For this review, use the dimensioned drawing (mm, ordinates from the lowest corner) and the shaded views. A direction names the side the tool comes from. Coordinates: 2 decimals unless noted, no trailing zeros. Order: outer loops, then holes, each group sorted by start corner. A loop starts at its lowest first (then second) coordinate and runs counter-clockwise, first axis right, second up. Notation, with made-up numbers: M 9.25,41.25 L 41.25,41.25 A18 cw 41.25,47.25 Z; hole C -8,65 d4. An arc over 180 degrees is marked long. One line per item, written item: value.
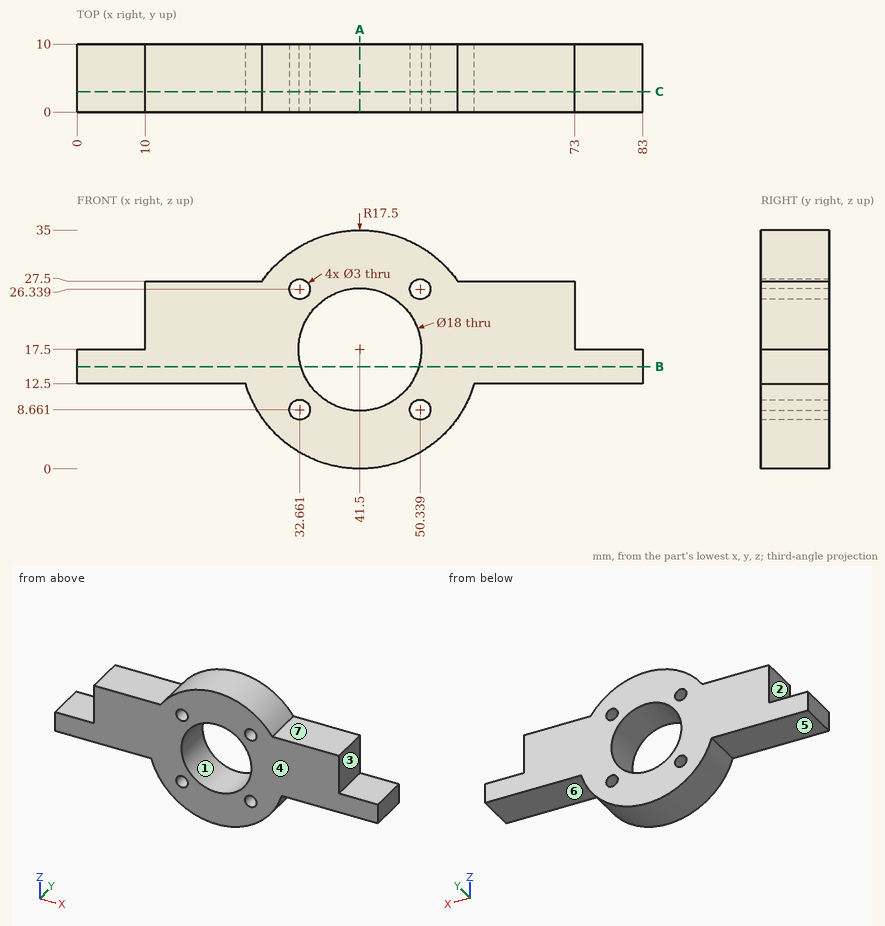
(1) For L1, parallel to X at y = 7.75, z = 17; L2, parallel to Z at x = 33.5, y = 1.5 (1 decimal); L3, parallel to Z at x = 67, y = 6.75, list the stretches that pass through material, from the lowest coordinate up.
Geometry results:
L1: x = 0 to 32.51, 50.49 to 83
L2: z = 1.9 to 7.4, 9.9 to 13.4, 21.6 to 25.1, 27.6 to 33.1
L3: z = 12.5 to 27.5
(2) We need section C-C, the plane y = 3. State the section outline as (x, z) points.
Geometry results:
outline: M 0,12.5 L 24.73,12.5 A17.5 ccw 58.27,12.5 L 83,12.5 L 83,17.5 L 73,17.5 L 73,27.5 L 55.86,27.5 A17.5 ccw 27.14,27.5 L 10,27.5 L 10,17.5 L 0,17.5 Z; hole C 32.66,8.66 d3; hole C 32.66,26.34 d3; hole C 41.5,17.5 d18; hole C 50.34,8.66 d3; hole C 50.34,26.34 d3
(3) We need section A-A, the plane x = 41.5. State the section outline as (y, z) points, plus the area to 3 significant figures.
Geometry results:
outline: M 0,0 L 10,0 L 10,8.5 L 0,8.5 Z; M 0,26.5 L 10,26.5 L 10,35 L 0,35 Z
area: 170 mm2
(4) Tool access review of the marked faces 5, 6 and 7: name each direction out of +Z, -Z, +X, -X, +Y, -Y from which nothing blocks a thin tool from reaching the whole face with its end or side.
Geometry results:
face 5: -Z, -X, +Y, -Y
face 6: -Z, +X, +Y, -Y
face 7: +Z, +X, +Y, -Y
(5) Insertion check: pin 1 Ø2 at (x, y) = (48.5, 6.5) entering from -Z; pin 2 Ø1.5 at (x, y) = (36, 3) entering from +Z; pin 3 Ø1.5 at (x, y) = (56.5, 6.5) entering from +Z. Each pin has a flat end and moves straight along its axis. Give the tip position at first contact, or say it passes through.
Geometry results:
pin 1: stops at z = 1.06
pin 2: stops at z = 34.34
pin 3: stops at z = 27.66
(6) We need section B-B, the plane z = 15. State the section outline as (x, y) points.
Geometry results:
outline: M 0,0 L 32.85,0 L 32.85,10 L 0,10 Z; M 50.15,0 L 83,0 L 83,10 L 50.15,10 Z
(7) Mouldability with a two-part tool opening along X and no side actions: class the marked faces 1, 2, 3 and 4 as +X half, -X half, draft (parallel to the pull), parting line (faces both ways), or undercut.
Geometry results:
face 1: undercut
face 2: -X half
face 3: +X half
face 4: draft
